```python
from build123d import *

# Parameters (mm, degrees)
SKETCH2_R           = 31.26
SKETCH2_W           = 400
SKETCH2_H           = 48.2
SKETCH2_W_2         = 1200
BOSS_EXTRUDE4_DEPTH = 10
SKETCH3_R           = 7.18
CUT_EXTRUDE1_DEPTH  = 10


with BuildPart() as part:
    # Sketch2 → Boss-Extrude4 (new body)
    with BuildSketch(Plane.XY):
        with Locations((400, -300)):
            Circle(SKETCH2_R)
        with Locations((800, -300)):
            Circle(SKETCH2_R)
        Circle(SKETCH2_R)
        with Locations((1200, 0)):
            Circle(SKETCH2_R)
        with Locations((600, -300)):
            Rectangle(SKETCH2_W, SKETCH2_H)
        with Locations((600, 0)):
            Rectangle(SKETCH2_W_2, SKETCH2_H)
        Polygon((414.610371201, -280.519505066), (14.610371201, 19.480494934), (-14.309628799, -19.079505066), (385.690371201, -319.079505066), align=None)
        Polygon((1185.687703452, 19.083062065), (785.687703452, -280.916937935), (814.607703452, -319.476937935), (1214.607703452, -19.476937935), align=None)
        Polygon((792.609480398, -319.708052273), (-7.390519602, -19.708052273), (9.533630282, 25.423014086), (809.533630282, -274.576985914), align=None)
    extrude(amount=BOSS_EXTRUDE4_DEPTH)

    # Sketch3 → Cut-Extrude1 (cut)
    with BuildSketch(Plane.XY.offset(10)):
        Circle(SKETCH3_R)
        with Locations((1200, 0)):
            Circle(SKETCH3_R)
        with Locations((800, -300)):
            Circle(SKETCH3_R)
        with Locations((400, -300)):
            Circle(SKETCH3_R)
    extrude(amount=-CUT_EXTRUDE1_DEPTH, mode=Mode.SUBTRACT)


solid = part.part
```
The model under review builds one solid part; all positions refer to its coordinate system, in mm. A direction names the side the tool comes from. Round coordinates to 2 decimals unless told otherwise and drop trailing zeros. Order: outer loops, then holes, each group sorted by start corner. A loop starts at its lowest first (then second) coordinate and runs counter-clockwise, first axis right, second up.
Item 1: Add section A-A, the plane z = 5. State the section outline as (x, y) points (3 decimals).
Working result:
outline: (1.857, -31.205) - (369.523, -306.954) arc R31.26 ccw to (419.909, -324.1) - (780.091, -324.1) arc R31.26 ccw to (830.294, -307.712) - (1198.922, -31.241) arc R31.26 ccw (long way) to (1180.091, 24.1) - (19.909, 24.1) arc R31.26 ccw (long way) to start; hole circle Ø14.36 at (0, 0); hole (141.114, -75.397) - (398.929, -268.758) arc R31.26 cw to (419.909, -275.9) - (675.788, -275.9) - close; hole (141.595, -24.1) - (795.029, -269.138) arc R31.26 cw to (801.851, -268.795) - (1128.11, -24.1) - close; hole circle Ø14.36 at (400, -300); hole circle Ø14.36 at (800, -300); hole circle Ø14.36 at (1200, 0)
Item 2: Add section D-D, the plane x = 854. State the section outline as (y, z) points, and give its area (3 significant figures).
Working result:
outline: (-289.93, 0) - (-229.68, 0) - (-229.68, 10) - (-289.93, 10) - close; (-24.1, 0) - (24.1, 0) - (24.1, 10) - (-24.1, 10) - close
area: 1,080 mm2
Item 3: Draft analysis for pull direction Y (two halves, no side actions). For faces 1 (the cylindrical face through (1229.855, 9.265, 4.93)), 2 (the flat face through (271.826, -173.431, 4.93)), 3 (the flat face through (1012.03, -171.41, 4.93)), state which applies: released by +Y, released by -Y, zero draft, split by the parting line, or undercut.
Working result:
face 1: split by the parting line
face 2: undercut
face 3: released by -Y
Item 4: For pin 1 (11.5 mm diameter, centred on x = 1200, y = 0, fed in from -Z); pin 2 (5 mm diameter, centred on x = 95.5, z = 7.5, fed in from +Y); pin 3 (3 mm diameter, centred on x = 838, z = 5.5, fed in from -Y), all flat-tipped, find the tip position at first contact; note any pin that passes through.
Working result:
pin 1: passes through
pin 2: stops at y = 24.1
pin 3: stops at y = -303.06
Item 5: Machinability: for faces 4 (the flat face through (967.264, -144.735, 4.93)), 5 (the flat face through (550, -189, 0)), which of the approach directions +Z, -Z, +X, -X, +Y, -Y give a long, thin tool a straight path to every point of the face, cutting with its end or side? Answer none if there is none.
Working result:
face 4: +Z, -Z
face 5: -Z, +X, -X, +Y, -Y
Item 6: Add section B-B, the plane y = -251. State the section outline as (x, z) points, and give its area (3 significant figures).
Working result:
outline: (294.92, 0) - (375.25, 0) - (375.25, 10) - (294.92, 10) - close; (609.39, 0) - (746.66, 0) - (746.66, 10) - (609.39, 10) - close; (825.58, 0) - (905.91, 0) - (905.91, 10) - (825.58, 10) - close
area: 2,980 mm2
Item 7: Add section C-C, the plane x = 437.5. State the section outline as (y, z) points, and give its area (3 significant figures).
Working result:
outline: (-324.1, 0) - (-275.9, 0) - (-275.9, 10) - (-324.1, 10) - close; (-186.54, 0) - (-135.06, 0) - (-135.06, 10) - (-186.54, 10) - close; (-24.1, 0) - (24.1, 0) - (24.1, 10) - (-24.1, 10) - close
area: 1,480 mm2
Item 8: To check wall thickness, follow probe 1 along Y at (x, z) = (800, 8); probe 2 along Y at (x, z) = (400, 2.25); probe 3 along X at (y, z) = (-300, 7.5). State the ranges of each line that lie inside material, in increasing order.
Working result:
probe 1: y = -331.26 to -307.18, -292.82 to -268.74, -24.1 to 24.1
probe 2: y = -331.26 to -307.18, -292.82 to -268.74, -172.48 to -121, -24.1 to 24.1
probe 3: x = 360.25 to 392.82, 407.18 to 792.82, 807.18 to 840.58
